Part model, mm, in its own coordinate system. A direction names the side the tool comes from. Round coordinates to 2 decimals unless told otherwise and drop trailing zeros. Order: outer loops, then holes, each group sorted by start corner. A loop starts at its lowest first (then second) coordinate and runs counter-clockwise, first axis right, second up. Notation, with made-up numbers: (73.5, 24) - (117.5, 24) arc R31 cw to (117.5, 50) - close; hole circle Ø5 at (58, 10.5). An arc over 180 degrees is marked (long way). Return JSON: item names as keys, results as strings. Group by question number.
Item 1: Probe probe 1 along Y at (x, z) = (15, 5.3); probe 2 along Y at (x, z) = (-22.7, 5.55); probe 3 along Z at (x, y) = (-10.5, -24.5). List the from-to ranges inside material, lowest first.
Item 2: Two-plate mould, pull along X, no slides. Class faces 3 (the face through (13.225, -23.899, 9.704)), 4 (the face through (-4, -40.5, 5)): released by +X, released by -X, zero draft, split by the parting line, or undercut.
Item 3: Tool access for faces 1 (the face through (13.8, -37.9, 4.9)), 2 (the face through (-8.025, -34.934, 9.704)): list every direction of +Z, -Z, +X, -X, +Y, -Y with a clear straight run to the whole face (end or side of a thin tool).
Item 4: Saw through at A-A on x = -22.7. List the corners of the cut face in (y, z).
Item 5: Saw through at C-C on x = -11. List the corners of the cut face in (y, z), and give its area (3 significant figures).
Item 6: Drop flat-ended pins along their axis: pin 1 (2 mm diameter, centred on x = -7, z = 8.5, fed in from -Y); pin 2 (1 mm diameter, centred on x = -1, y = -10.5, fed in from +Z); pin 3 (1.5 mm diameter, centred on y = -24.5, z = 10.5, fed in from -X); pin 4 (2.5 mm diameter, centred on x = 15, y = -37, fed in from +Z). Give the stop position or say it passes through.
```python
from build123d import *

# Parameters (mm, degrees)
SKETCH011_W                   = 44.7
SKETCH011_H                   = 44.7
PAD006_DEPTH                  = 3.3
FILLET001_R                   = 0.5
PAD007_DEPTH                  = 6.5
PAD007_LINEARPATTERN_2_DEPTH  = 6.5
PAD007_LINEARPATTERN_3_DEPTH  = 6.5
PAD007_LINEARPATTERN_4_DEPTH  = 6.5
PAD007_LINEARPATTERN_5_DEPTH  = 6.5
PAD007_LINEARPATTERN_6_DEPTH  = 6.5
PAD007_LINEARPATTERN_7_DEPTH  = 6.5
PAD007_LINEARPATTERN_8_DEPTH  = 6.5
PAD007_LINEARPATTERN_9_DEPTH  = 6.5
PAD007_LINEARPATTERN_10_DEPTH = 6.5
PAD007_LINEARPATTERN_11_DEPTH = 6.5
LINEARPATTERN001_COUNT        = 4
LINEARPATTERN001_PITCH        = 11.1666666667
SKETCH013_W                   = 4.44947025
SKETCH013_H                   = 9.881485
POCKET006_DEPTH               = 6.5
SKETCH014_W                   = 4.44947025
SKETCH014_H                   = 9.4
POCKET007_DEPTH               = 6.5
SKETCH015_R                   = 1.5
POCKET008_DEPTH               = 3.301


with BuildPart() as part:
    # Sketch011 → Pad006 (new body)
    with BuildSketch(Plane.XY):
        with Locations((-3.85, -18.15)):
            Rectangle(SKETCH011_W, SKETCH011_H)
    extrude(amount=PAD006_DEPTH)

    # Fillet001
    fillet001_edges = [part.edges().sort_by_distance(p)[0] for p in [
        (-3.85, 4.2, 3.3),
        (-26.2, -18.15, 3.3),
        (18.5, -18.15, 3.3),
        (-3.85, -40.5, 3.3),
        (-26.2, 4.2, 1.65),
        (-26.2, -40.5, 1.65),
        (18.5, 4.2, 1.65),
        (18.5, -40.5, 1.65),
    ]]
    fillet(fillet001_edges, radius=FILLET001_R)

    # Sketch012 (on Face13 of Fillet001) → Pad007 (join)
    with BuildSketch(Plane.XY.offset(3.3)):
        with BuildLine():
            ThreePointArc((-24.7, -6.2), (-24.575264875, -1.5), (-24.7, 3.2))
            ThreePointArc((-24.7, 3.2), (-24.824735125, -1.5), (-24.7, -6.2))
        make_face()
    pad007 = extrude(amount=PAD007_DEPTH)

    # Sketch012 LinearPattern 2 → Pad007 LinearPattern 2 (add)
    with BuildSketch(Plane(origin=(4.2, 0, 3.3), x_dir=(1, 0, 0), z_dir=(0, 0, 1))):
        with BuildLine():
            ThreePointArc((-24.7, -6.2), (-24.575264875, -1.5), (-24.7, 3.2))
            ThreePointArc((-24.7, 3.2), (-24.824735125, -1.5), (-24.7, -6.2))
        make_face()
    pad007_linearpattern_2 = extrude(amount=PAD007_LINEARPATTERN_2_DEPTH)

    # Sketch012 LinearPattern 3 → Pad007 LinearPattern 3 (add)
    with BuildSketch(Plane(origin=(8.4, 0, 3.3), x_dir=(1, 0, 0), z_dir=(0, 0, 1))):
        with BuildLine():
            ThreePointArc((-24.7, -6.2), (-24.575264875, -1.5), (-24.7, 3.2))
            ThreePointArc((-24.7, 3.2), (-24.824735125, -1.5), (-24.7, -6.2))
        make_face()
    pad007_linearpattern_3 = extrude(amount=PAD007_LINEARPATTERN_3_DEPTH)

    # Sketch012 LinearPattern 4 → Pad007 LinearPattern 4 (add)
    with BuildSketch(Plane(origin=(12.6, 0, 3.3), x_dir=(1, 0, 0), z_dir=(0, 0, 1))):
        with BuildLine():
            ThreePointArc((-24.7, -6.2), (-24.575264875, -1.5), (-24.7, 3.2))
            ThreePointArc((-24.7, 3.2), (-24.824735125, -1.5), (-24.7, -6.2))
        make_face()
    pad007_linearpattern_4 = extrude(amount=PAD007_LINEARPATTERN_4_DEPTH)

    # Sketch012 LinearPattern 5 → Pad007 LinearPattern 5 (add)
    with BuildSketch(Plane(origin=(16.8, 0, 3.3), x_dir=(1, 0, 0), z_dir=(0, 0, 1))):
        with BuildLine():
            ThreePointArc((-24.7, -6.2), (-24.575264875, -1.5), (-24.7, 3.2))
            ThreePointArc((-24.7, 3.2), (-24.824735125, -1.5), (-24.7, -6.2))
        make_face()
    pad007_linearpattern_5 = extrude(amount=PAD007_LINEARPATTERN_5_DEPTH)

    # Sketch012 LinearPattern 6 → Pad007 LinearPattern 6 (add)
    with BuildSketch(Plane(origin=(21, 0, 3.3), x_dir=(1, 0, 0), z_dir=(0, 0, 1))):
        with BuildLine():
            ThreePointArc((-24.7, -6.2), (-24.575264875, -1.5), (-24.7, 3.2))
            ThreePointArc((-24.7, 3.2), (-24.824735125, -1.5), (-24.7, -6.2))
        make_face()
    pad007_linearpattern_6 = extrude(amount=PAD007_LINEARPATTERN_6_DEPTH)

    # Sketch012 LinearPattern 7 → Pad007 LinearPattern 7 (add)
    with BuildSketch(Plane(origin=(25.2, 0, 3.3), x_dir=(1, 0, 0), z_dir=(0, 0, 1))):
        with BuildLine():
            ThreePointArc((-24.7, -6.2), (-24.575264875, -1.5), (-24.7, 3.2))
            ThreePointArc((-24.7, 3.2), (-24.824735125, -1.5), (-24.7, -6.2))
        make_face()
    pad007_linearpattern_7 = extrude(amount=PAD007_LINEARPATTERN_7_DEPTH)

    # Sketch012 LinearPattern 8 → Pad007 LinearPattern 8 (add)
    with BuildSketch(Plane(origin=(29.4, 0, 3.3), x_dir=(1, 0, 0), z_dir=(0, 0, 1))):
        with BuildLine():
            ThreePointArc((-24.7, -6.2), (-24.575264875, -1.5), (-24.7, 3.2))
            ThreePointArc((-24.7, 3.2), (-24.824735125, -1.5), (-24.7, -6.2))
        make_face()
    pad007_linearpattern_8 = extrude(amount=PAD007_LINEARPATTERN_8_DEPTH)

    # Sketch012 LinearPattern 9 → Pad007 LinearPattern 9 (add)
    with BuildSketch(Plane(origin=(33.6, 0, 3.3), x_dir=(1, 0, 0), z_dir=(0, 0, 1))):
        with BuildLine():
            ThreePointArc((-24.7, -6.2), (-24.575264875, -1.5), (-24.7, 3.2))
            ThreePointArc((-24.7, 3.2), (-24.824735125, -1.5), (-24.7, -6.2))
        make_face()
    pad007_linearpattern_9 = extrude(amount=PAD007_LINEARPATTERN_9_DEPTH)

    # Sketch012 LinearPattern 10 → Pad007 LinearPattern 10 (add)
    with BuildSketch(Plane(origin=(37.8, 0, 3.3), x_dir=(1, 0, 0), z_dir=(0, 0, 1))):
        with BuildLine():
            ThreePointArc((-24.7, -6.2), (-24.575264875, -1.5), (-24.7, 3.2))
            ThreePointArc((-24.7, 3.2), (-24.824735125, -1.5), (-24.7, -6.2))
        make_face()
    pad007_linearpattern_10 = extrude(amount=PAD007_LINEARPATTERN_10_DEPTH)

    # Sketch012 LinearPattern 11 → Pad007 LinearPattern 11 (add)
    with BuildSketch(Plane(origin=(42, 0, 3.3), x_dir=(1, 0, 0), z_dir=(0, 0, 1))):
        with BuildLine():
            ThreePointArc((-24.7, -6.2), (-24.575264875, -1.5), (-24.7, 3.2))
            ThreePointArc((-24.7, 3.2), (-24.824735125, -1.5), (-24.7, -6.2))
        make_face()
    pad007_linearpattern_11 = extrude(amount=PAD007_LINEARPATTERN_11_DEPTH)

    # LinearPattern001: Pad007, Pad007 LinearPattern 2, Pad007 LinearPattern 3, Pad007 LinearPattern 4, Pad007 LinearPattern 5, Pad007 LinearPattern 6, Pad007 LinearPattern 7, Pad007 LinearPattern 8, Pad007 LinearPattern 9, Pad007 LinearPattern 10, Pad007 LinearPattern 11 ×4
    with Locations(*[(0, -i * LINEARPATTERN001_PITCH, 0) for i in range(1, LINEARPATTERN001_COUNT)]):
        add(pad007)
        add(pad007_linearpattern_2)
        add(pad007_linearpattern_3)
        add(pad007_linearpattern_4)
        add(pad007_linearpattern_5)
        add(pad007_linearpattern_6)
        add(pad007_linearpattern_7)
        add(pad007_linearpattern_8)
        add(pad007_linearpattern_9)
        add(pad007_linearpattern_10)
        add(pad007_linearpattern_11)

    # Sketch013 (on Face147 of MultiTransform001) → Pocket006 (cut)
    with BuildSketch(Plane.XY.offset(9.8)):
        with Locations((-22.6, -1.7407425)):
            Rectangle(SKETCH013_W, SKETCH013_H)
    extrude(amount=-POCKET006_DEPTH, mode=Mode.SUBTRACT)

    # Sketch014 (on Face125 of Pocket006) → Pocket007 (cut)
    with BuildSketch(Plane.XY.offset(9.8)):
        with Locations((15.2, -35)):
            Rectangle(SKETCH014_W, SKETCH014_H)
    extrude(amount=-POCKET007_DEPTH, mode=Mode.SUBTRACT)

    # Sketch015 (on Face13 of Pocket007) → Pocket008 (cut, through all)
    with BuildSketch(Plane.XY.offset(3.3)):
        with Locations((-22.7, 0.7)):
            Circle(SKETCH015_R)
        with Locations((15, -37)):
            Circle(SKETCH015_R)
    extrude(amount=-POCKET008_DEPTH, mode=Mode.SUBTRACT)


with BuildPart() as part_1:
    # Body002 placement: moved
    add(part.part.moved(Location((0, 0, 3.2))))


solid = part_1.part
```
Filled in:
{
 "1": {"probe 1": "y = -40.5 to -38.5, -35.5 to 4.2", "probe 2": "y = -40.5 to -0.8, 2.2 to 4.2", "probe 3": "z = 3.2 to 6.5"},
 "2": {"face 3": "undercut", "face 4": "zero draft"},
 "3": {"face 1": "+Z, -Z", "face 2": "+Z"},
 "4": {"outline": "(-40.5, 3.2) - (-0.8, 3.2) - (-0.8, 6.5) - (-40, 6.5) arc R0.5 ccw to (-40.5, 6) - close; (2.2, 3.2) - (4.2, 3.2) - (4.2, 6) arc R0.5 ccw to (3.7, 6.5) - (2.2, 6.5) - close"},
 "5": {"outline": "(-40.5, 3.2) - (4.2, 3.2) - (4.2, 6) arc R0.5 ccw to (3.7, 6.5) - (-40, 6.5) arc R0.5 ccw to (-40.5, 6) - close", "area": "147 mm^2"},
 "6": {"pin 1": "stops at y = -39.7", "pin 2": "stops at z = 6.5", "pin 3": "stops at x = -24.82", "pin 4": "passes through"}
}
